from build123d import *

# Parameters (mm, degrees)
F0_W     = 152.4
F0_H     = 101.6
F1_DEPTH = 12.7
F3_DEPTH = 50.8
F4_R     = 5.08
F5_R     = 5.08
F6_R     = 5.08
F7_R     = 5.08
F8_R     = 26.410315
F9_DEPTH = 63.501
F10_SIZE = 5.08


with BuildPart() as f1:
    # F0 (on Front) → F1 (new body)
    with BuildSketch(Plane.XZ):
        Rectangle(F0_W, F0_H)
    extrude(amount=F1_DEPTH)

    # F2 (on face) → F3 (join)
    with BuildSketch(Plane.XZ.offset(12.7)):
        Polygon((33.02, 50.8), (-33.02, 50.8), (-33.02, 0), (-58.42, 0), (-58.42, -50.8), (-38.1, -50.8), (-38.1, -25.4), (38.1, -25.4), (38.1, -50.8), (58.42, -50.8), (58.42, 0), (33.02, 0), align=None)
    extrude(amount=F3_DEPTH)

    # F4
    f4_edges = [f1.edges().sort_by_distance(p)[0] for p in [
        (76.2, -6.35, 50.8),
    ]]
    fillet(f4_edges, radius=F4_R)

    # F5
    f5_edges = [f1.edges().sort_by_distance(p)[0] for p in [
        (-76.2, -6.35, 50.8),
    ]]
    fillet(f5_edges, radius=F5_R)

    # F6
    f6_edges = [f1.edges().sort_by_distance(p)[0] for p in [
        (33.02, -38.1, 0),
    ]]
    fillet(f6_edges, radius=F6_R)

    # F7
    f7_edges = [f1.edges().sort_by_distance(p)[0] for p in [
        (-33.02, -38.1, 0),
    ]]
    fillet(f7_edges, radius=F7_R)

    # F8 (on Front) → F9 (cut, through all)
    with BuildSketch(Plane.XZ):
        with Locations((0, 50.8)):
            Circle(F8_R)
    extrude(amount=F9_DEPTH, mode=Mode.SUBTRACT)

    # F10
    f10_edges = [f1.edges().sort_by_distance(p)[0] for p in [
        (0, -63.5, -25.4),
        (-38.1, -63.5, -38.1),
        (38.1, -63.5, -38.1),
    ]]
    chamfer(f10_edges, length=F10_SIZE)


solid = f1.part
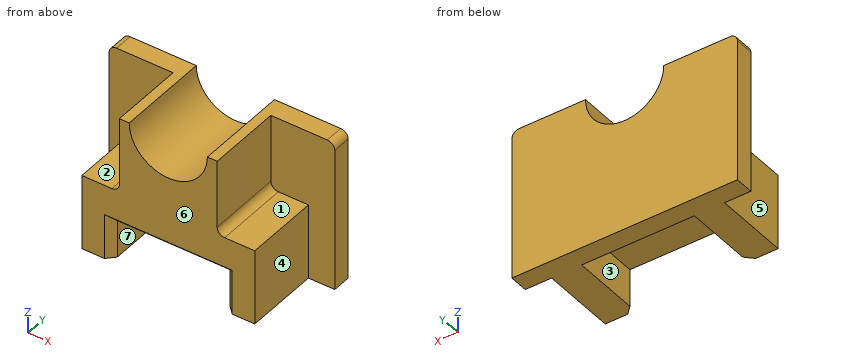
Model file for the job. Use its own axes, mm. Face numbers are marked on the shaded views. A direction names the side the tool comes from. Coordinates: 2 decimals unless noted, no trailing zeros. Loops run counter-clockwise (first coordinate to the right, second up) from the corner with the lowest first, then second, coordinate; pieces in that order, holes last. Notation, with made-up numbers: (39, -26) -> (93, -26) arc R15 ccw to (93, -12) -> close; hole circle Ø3 at (74, -28.75). An arc over 180 degrees is marked (long way). Use one line per item in the form item = value. Start each with the question number.
(1) Cut at B-B on z = 13.5. Give the cut face in (x, y).
(2) Pull direction X, two halves, no side cores. Call the marked faces 4, 5, 6 and 7: pulls with the +X half, pulls with the -X half, needs draft (parallel to the pull), parting line crosses it, or undercut.
(3) Probe probe 1 along X at (y, z) = (-46, -28); probe 2 along Z at (x, y) = (-0.5, -48); probe 3 along Y at (x, z) = (-67.5, 8). List the from-to ranges inside material, lowest first. Write a range as from..to.
(4) Cut at A-A on x = 0. Give the cut face in (y, z), and give its area (3 significant figures).
(5) Flat gauge pins, fed straight in: pin 1 (12 mm diameter, centred on y = -33, z = -13.5, fed in from -X); pin 2 (12.5 mm diameter, centred on y = -27, z = -42.5, fed in from +X); pin 3 (1.5 mm diameter, centred on y = -39.5, z = 3.5, fed in from +X); pin 4 (6 mm diameter, centred on x = -11, z = 32, fed in from -Y). Where does each tip first touch, or does it go through?
(6) Cut at D-D on x = -41. Give the cut face in (y, z), and give its area (3 significant figures).
(7) Tool access for the marked faces 1, 2 and 3: list every direction of +Z, -Z, +X, -X, +Y, -Y with a clear straight run to the whole face (end or side of a thin tool).
(8) Cut at C-C on z = 31. Give the cut face in (x, y).
Values:
q1.outline = (-76.2, -12.7) -> (-33.02, -12.7) -> (-33.02, -63.5) -> (33.02, -63.5) -> (33.02, -12.7) -> (76.2, -12.7) -> (76.2, 0) -> (-76.2, 0) -> close
q2.face_4 = pulls with the +X half
q2.face_5 = pulls with the -X half
q2.face_6 = needs draft
q2.face_7 = undercut
q3.probe_1 = -58.42..-38.1, 38.1..58.42
q3.probe_2 = -25.4..24.39
q3.probe_3 = -12.7..0
q4.outline = (-63.5, -20.32) -> (-58.42, -25.4) -> (-12.7, -25.4) -> (-12.7, -50.8) -> (0, -50.8) -> (0, 24.39) -> (-63.5, 24.39) -> close
q4.area = 3,470 mm2
q5.pin_1 = -58.42
q5.pin_2 = 58.42
q5.pin_3 = 33.59
q5.pin_4 = through
q6.outline = (-63.5, -20.32) -> (-61.32, -22.5) -> (-61.32, -50.8) -> (0, -50.8) -> (0, 50.8) -> (-12.7, 50.8) -> (-12.7, 0) -> (-63.5, 0) -> close
q6.area = 3,810 mm2
q7.face_1 = +Z, +X, -Y
q7.face_2 = +Z, -X, -Y
q7.face_3 = -Z, -Y
q8.outline = (-76.2, -12.7) -> (-33.02, -12.7) -> (-33.02, -63.5) -> (-17.48, -63.5) -> (-17.48, 0) -> (-76.2, 0) -> close; (17.48, -63.5) -> (33.02, -63.5) -> (33.02, -12.7) -> (76.2, -12.7) -> (76.2, 0) -> (17.48, 0) -> close
